```python
from build123d import *

# Parameters (mm, degrees)
F0_R     = 2.5
F1_DEPTH = 30
F3_R     = 5
F4_DEPTH = 6
F7_DEPTH = 5


with BuildPart() as f1:
    # F0 (on Front) → F1 (new body)
    with BuildSketch(Plane.XZ):
        Circle(F0_R)
    extrude(amount=-F1_DEPTH)

    # F3 (on offset) → F4 (join)
    with BuildSketch(Plane.XZ):
        Circle(F3_R)
    extrude(amount=F4_DEPTH)

    # F6 (on offset) → F7 (cut)
    with BuildSketch(Plane.XZ.offset(6)):
        Polygon((1.5, 2.598076), (-1.5, 2.598076), (-3, 0), (-1.5, -2.598076), (1.5, -2.598076), (3, 0), align=None)
    extrude(amount=-F7_DEPTH, mode=Mode.SUBTRACT)


solid = f1.part
```
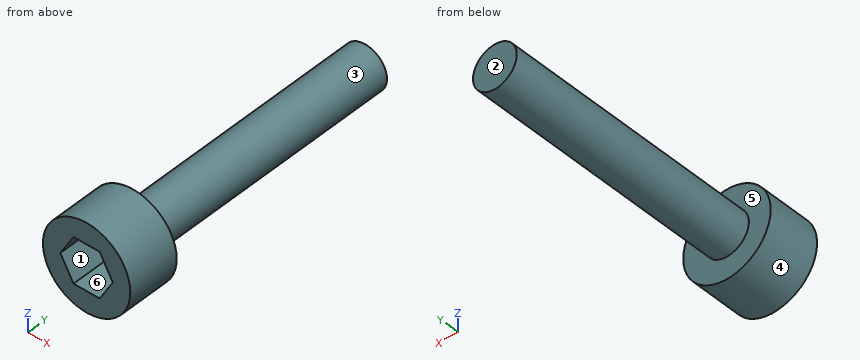
Model file for the job. Use its own axes, mm. Face numbers are marked on the shaded views. A direction names the side the tool comes from. Coordinates: 2 decimals unless noted, no trailing zeros. Write each loop counter-clockwise with the first axis right and the second up, starting at its lowest first coordinate (ties: lowest second). Pieces come first, ordered by that corner, then holes. Notation, with made-up numbers: (-5.75, 45.25) - (19.25, 45.25) arc R28 cw to (19.25, 81.25) - close; hole circle Ø7 at (53, 62.5). An arc over 180 degrees is marked (long way). Use a Markdown table: item, result. Add a question column.
Item 1: Two-plate mould, pull along Z, no slides. Class the marked faces 4, 5 and 6: pulls with the +Z half, pulls with the -Z half, needs draft (parallel to the pull), parting line crosses it, or undercut.
Item 2: Drill centre lines: line 1 along X through (y, z) = (-1.5, -4); line 2 along Y through (x, z) = (-0.25, -4.5); line 3 along Z through (x, y) = (2, 13.5). Where is each one in solid material? Low to high.
Item 3: Band-saw the part on C-C, the plane y = 5. Write the cut outline in (x, z).
Item 4: Drop flat-ended pins along their axis: pin 1 (0.9 mm diameter, centred on x = -0.5, y = -3.5, fed in from +Z); pin 2 (1 mm diameter, centred on x = 3, z = 2, fed in from +Y); pin 3 (4 mm diameter, centred on x = 0, z = 0.5, fed in from -Y); pin 4 (4 mm diameter, centred on y = 10, z = -0.5, fed in from -X). Give the stop position or say it passes through.
Item 5: Band-saw the part on D-D, the plane x = -4. Write the cut outline in (y, z), and give its area (3 significant figures).
Item 6: Band-saw the part on B-B, the plane x = 0. Write the cut outline in (y, z).
Item 7: Band-saw the part on A-A, the plane z = -2. Write the cut outline in (x, y).
Item 8: 3-axis set-ups, long thin cutter, end or side, ignore diameter. For the marked faces 1, 2 and 3: which of +Z, -Z, +X, -X, +Y, -Y reach the whole face in a straight line?
A:
| question | item | result |
|---|---|---|
| 1 | face 4 | parting line crosses it |
| 1 | face 5 | needs draft |
| 1 | face 6 | undercut |
| 2 | line 1 | x = -3 to 3 |
| 2 | line 2 | y = -6 to 0 |
| 2 | line 3 | z = -1.5 to 1.5 |
| 3 | outline | circle Ø5 at (0, 0) |
| 4 | pin 1 | stops at z = 5 |
| 4 | pin 2 | stops at y = 0 |
| 4 | pin 3 | stops at y = -1 |
| 4 | pin 4 | stops at x = -2.5 |
| 5 | outline | (-6, -3) - (0, -3) - (0, 3) - (-6, 3) - close |
| 5 | area | 36.0 mm² |
| 6 | outline | (-6, -5) - (0, -5) - (0, -2.5) - (30, -2.5) - (30, 2.5) - (0, 2.5) - (0, 5) - (-6, 5) - (-6, 2.6) - (-1, 2.6) - (-1, -2.6) - (-6, -2.6) - close |
| 7 | outline | (-4.58, -6) - (-1.85, -6) - (-1.85, -1) - (1.85, -1) - (1.85, -6) - (4.58, -6) - (4.58, 0) - (1.5, 0) - (1.5, 30) - (-1.5, 30) - (-1.5, 0) - (-4.58, 0) - close |
| 8 | face 1 | -Y |
| 8 | face 2 | +Z, -Z, +X, -X, +Y |
| 8 | face 3 | +Y |
